```python
from build123d import *

# Parameters (mm, degrees)
BOSS_EXTRUDE1_DEPTH      = 2.54
BOSS_EXTRUDE4_DEPTH      = 25.4
BOSS_EXTRUDE4_DEPTH_BACK = 12.7


with BuildPart() as part:
    # Sketch1 → Boss-Extrude1 (new body)
    with BuildSketch(Plane(origin=(0, 0, 0), x_dir=(1, 0, 0), z_dir=(0, 1, 0))):
        Polygon((-6.35, 69.85), (6.35, 69.85), (6.35, 6.35), (69.85, 6.35), (69.85, -6.35), (-6.35, -6.35), align=None)
    extrude(amount=BOSS_EXTRUDE1_DEPTH)

    # Sketch2 → Boss-Extrude4 (add, two sides: drawn at the far end of the back side and taken through both)
    with BuildSketch(Plane(origin=(0, 2.54, 0), x_dir=(1, 0, 0), z_dir=(0, 1, 0)).offset(-BOSS_EXTRUDE4_DEPTH_BACK)):
        with BuildLine():
            Line((-18.900260769, 70.536733465), (-18.0785103, 67.469918966))
            ThreePointArc((-18.0785103, 67.469918966), (49.391408666, 49.391408666), (67.469918966, -18.0785103))
            Line((67.469918966, -18.0785103), (70.536733465, -18.900260769))
            ThreePointArc((70.536733465, -18.900260769), (51.636472696, 51.636472696), (-18.900260769, 70.536733465))
        make_face()
    extrude(amount=BOSS_EXTRUDE4_DEPTH + BOSS_EXTRUDE4_DEPTH_BACK)


solid = part.part
```
Geometry check sheet. Reference: the model listing, model coordinates, mm. A direction names the side the tool comes from. Give positions to 0.01 mm unless a question says otherwise; leave off trailing zeros. Order: outer loops, then holes, each group sorted by start corner. A loop starts at its lowest first (then second) coordinate and runs counter-clockwise, first axis right, second up. Notation, with made-up numbers: (-14, 8.5) - (13, 8.5) arc R20 cw to (13, 18.5) - close; hole circle Ø3 at (59.25, -40). An arc over 180 degrees is marked (long way). Write item = value, one per line. Start each with the question number.
1) Section check C-C (z = -3). Enter the section's corners in (x, y), then the cut area to 3 significant figures.
2) Draft check along Z on faces 3 (the flat face through (-18.495, 8.623, -69.025)), 4 (the flat face through (44, -10.16, -55)), 5 (the flat face through (6.35, 1, -38)). Enter one of: released by +Z, released by -Z, zero draft, split by the parting line, or undercut.
3) Scan lines: L1, parallel to X at y = 1.5, z = -32; L2, parallel to Y at x = 34, z = 1.5; L3, parallel to Z at x = 53, y = 7. Record each from-to range of solid material in increasing order.
4) Section check D-D (y = 10.5). Enter the section's corners in (x, z) (3 decimals).
5) Section check B-B (x = 66). Enter the section's corners in (y, z).
6) Access from +Z, -Z, +X, -X, +Y, -Y to the whole of each face (thin tool, end or side, straight path). Record for faces 1 (the flat face through (38, 1, -6.35)), 2 (the flat face through (44, 27.94, -55)).
7) Section check A-A (z = -52). Enter the section's corners in (x, y).
8) Gauge pin test, flat ends, axial feed: pin 1 Ø2 at (y, z) = (2, -48.5) entering from +X; pin 2 Ø10 at (y, z) = (17, -18.5) entering from -X; pin 3 Ø3 at (x, y) = (40, 4.5) entering from +Z. Record the tip position at first contact, or that the pin passes through.
Geometry check:
q1.outline = (-6.35, 0) - (69.79, 0) - (69.79, -10.16) - (72.96, -10.16) - (72.96, 27.94) - (69.79, 27.94) - (69.79, 2.54) - (-6.35, 2.54) - close
q1.area = 314 mm2
q2.face_3 = released by +Z
q2.face_4 = zero draft
q2.face_5 = undercut
q3.L1 = -6.35 to 6.35, 62.09 to 65.64
q3.L2 = 0 to 2.54
q3.L3 = -50.24 to -45.5
q4.outline = (-18.9, -70.537) arc R73.025 ccw to (70.537, 18.9) - (67.47, 18.079) arc R69.85 cw to (-18.079, -67.47) - close
q5.outline = (-10.16, -31.25) - (27.94, -31.25) - (27.94, -22.87) - (-10.16, -22.87) - close; (0, -6.35) - (2.54, -6.35) - (2.54, 6.35) - (0, 6.35) - close
q6.face_1 = +Y, -Y
q6.face_2 = +Z, -Z, +X, -X, +Y
q7.outline = (-6.35, 0) - (6.35, 0) - (6.35, 2.54) - (-6.35, 2.54) - close; (46.64, -10.16) - (51.27, -10.16) - (51.27, 27.94) - (46.64, 27.94) - close
q8.pin_1 = 55.47
q8.pin_2 = 65.78
q8.pin_3 = -56.19
